```python
from build123d import *

# Parameters (mm, degrees)
SKICA1_W                = 55
SKICA1_H                = 30
P_IDAT_VYSUNUT_M1_DEPTH = 7
ZAOBLIT1_R              = 10
SKO_EPINA1_T            = -1.6


with BuildPart() as part:
    # Skica1 → Přidat vysunutím1 (new body)
    with BuildSketch(Plane(origin=(0, 0, 0), x_dir=(1, 0, 0), z_dir=(0, 1, 0))):
        with Locations((-27.5, 15)):
            Rectangle(SKICA1_W, SKICA1_H)
    extrude(amount=P_IDAT_VYSUNUT_M1_DEPTH)

    # Zaoblit1
    zaoblit1_edges = [part.edges().sort_by_distance(p)[0] for p in [
        (0, 3.5, 0),
        (-55, 3.5, 0),
        (-55, 3.5, -30),
        (0, 3.5, -30),
    ]]
    fillet(zaoblit1_edges, radius=ZAOBLIT1_R)

    # Skořepina1
    sko_epina1_openings = [part.faces().sort_by_distance(p)[0] for p in [
        (-27.5, 7, -15),
    ]]
    offset(amount=SKO_EPINA1_T, openings=sko_epina1_openings, kind=Kind.INTERSECTION)


solid = part.part
```
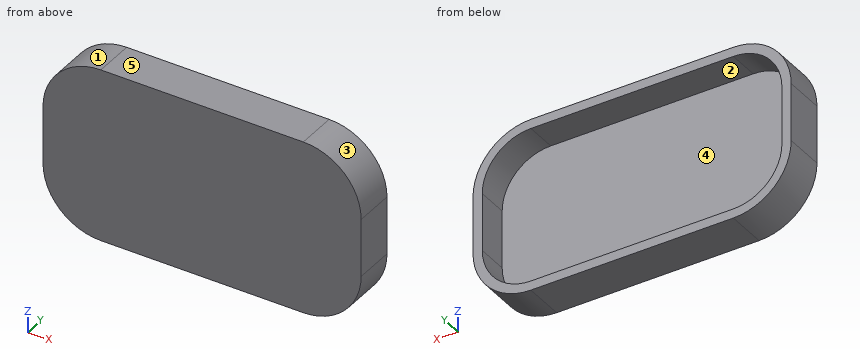
Check sheet for the modelled part. Datum: model origin and axes. Units: mm. Face numbers are marked on the shaded views. A direction names the side the tool comes from. Give positions to 0.01 mm unless a question says otherwise; leave off trailing zeros. Order: outer loops, then holes, each group sorted by start corner. A loop starts at its lowest first (then second) coordinate and runs counter-clockwise, first axis right, second up. Notation, with made-up numbers: M -37,32 L 20,32 A25 ccw 20,56 Z; hole C 33,5 d6. An arc over 180 degrees is marked long. Answer in a Markdown table with one row per item. Add a question column.
Q1. Access from +Z, -Z, +X, -X, +Y, -Y to the whole of each face (thin tool, end or side, straight path). Record for the marked faces 4 and 5.
Q2. Release check for a two-part mould opening along X. For the marked faces 1, 2 and 3 record: released by +X, released by -X, zero draft, split by the parting line, or undercut.
Q3. Sectioned sample at C-C, the plane x = -19. Record the boundary of the cut face in (y, z), and give its area (3 significant figures).
Q4. Thickness scan on L1, parallel to X at y = 3, z = -10.25; L2, parallel to Z at x = -23, y = 3.25; L3, parallel to Y at x = -24, z = -20.5. Record the ranges inside material, lowest first.
Q5. Sectioned sample at B-B, the plane z = -13.5. Record the boundary of the cut face in (x, y).
Q6. Gauge pin test, flat end, axial feed: pin 1 Ø8 at (x, z) = (-43.5, -21.5) entering from +Y. Record the tip position at first contact, or that the pin passes through.
Q7. Sectioned sample at A-A, the plane y = 3.5. Record the boundary of the cut face in (x, z), and give its area (3 significant figures).
Verdict:
| question | item | result |
|---|---|---|
| 1 | face 4 | +Y |
| 1 | face 5 | +Z, +X, -X, +Y, -Y |
| 2 | face 1 | released by -X |
| 2 | face 2 | undercut |
| 2 | face 3 | released by +X |
| 3 | outline | M 0,-30 L 7,-30 L 7,-28.4 L 1.6,-28.4 L 1.6,-1.6 L 7,-1.6 L 7,0 L 0,0 Z |
| 3 | area | 65.3 mm² |
| 4 | L1 | -55 to -53.4, -1.6 to 0 |
| 4 | L2 | -30 to -28.4, -1.6 to 0 |
| 4 | L3 | 0 to 1.6 |
| 5 | outline | M -55,0 L 0,0 L 0,7 L -1.6,7 L -1.6,1.6 L -53.4,1.6 L -53.4,7 L -55,7 Z |
| 6 | pin 1 | y = 1.6 |
| 7 | outline | M -55,-20 A10 ccw -45,-30 L -10,-30 A10 ccw 0,-20 L 0,-10 A10 ccw -10,0 L -45,0 A10 ccw -55,-10 Z; hole M -53.4,-20 A8.4 ccw -45,-28.4 L -10,-28.4 A8.4 ccw -1.6,-20 L -1.6,-10 A8.4 ccw -10,-1.6 L -45,-1.6 A8.4 ccw -53.4,-10 Z |
| 7 | area | 236 mm² |
